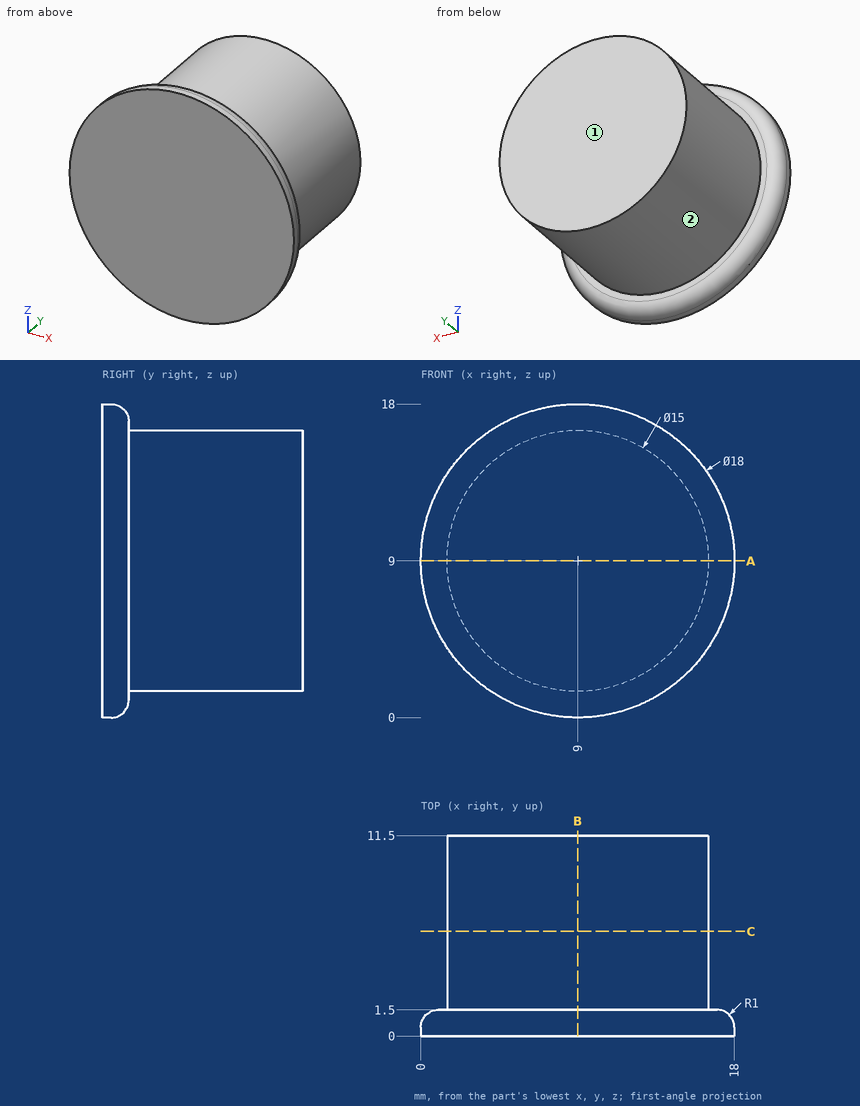
Check sheet for the drawn part. Datum: minimum x, y, z corner. Units: mm. A direction names the side the tool comes from. Round coordinates to 2 decimals unless told otherwise and drop trailing zeros. Write each loop counter-clockwise with the first axis right and the second up, starting at its lowest first coordinate (ties: lowest second). Pieces come first, ordered by that corner, then holes. Notation, with made-up numbers: (2, 86.25) -> (36, 86.25) arc R10 cw to (36, 93.25) -> close; hole circle Ø5 at (-6, -30.75). An arc over 180 degrees is marked (long way). One line per item, written item: value. Start each with the question number.
(1) Scan lines: line 1 (Z direction, x = 15.25, y = 3); line 2 (X direction, y = 8.75, z = 13); line 3 (Z direction, x = 4.75, y = 4). Record each from-to range of solid material in increasing order. Write a range as [from, to].
(2) Cross-section at C-C, the plane y = 6. Record the cut outline in (x, z).
(3) Go/stop test with flat-tipped pins: pin 1 Ø2 at (y, z) = (1.5, 13) entering from +X; pin 2 Ø1 at (y, z) = (6, 4) entering from +X; pin 3 Ø1.5 at (y, z) = (6, 2) entering from +X. Record where each tip stops, or that it passes through.
(4) Cross-section at B-B, the plane x = 9. Record the cut outline in (y, z), and give its area (3 significant figures).
(5) Access from +Z, -Z, +X, -X, +Y, -Y to the whole of each face (thin tool, end or side, straight path). Record for the marked faces 1 and 2.
(6) Cross-section at A-A, the plane z = 9. Record the cut outline in (x, y), and give its area (3 significant figures).
Answer:
1. line 1: [4.85, 13.15]
1. line 2: [2.66, 15.34]
1. line 3: [2.82, 15.18]
2. outline: circle Ø15 at (9, 9)
3. pin 1: x = 17.33
3. pin 2: x = 15
3. pin 3: x = 13.15
4. outline: (0, 0) -> (0.5, 0) arc R1 ccw to (1.5, 1) -> (1.5, 1.5) -> (11.5, 1.5) -> (11.5, 16.5) -> (1.5, 16.5) -> (1.5, 17) arc R1 ccw to (0.5, 18) -> (0, 18) -> close
4. area: 177 mm²
5. face 1: +Z, -Z, +X, -X, +Y
5. face 2: +Y
6. outline: (0, 0) -> (18, 0) -> (18, 0.5) arc R1 ccw to (17, 1.5) -> (16.5, 1.5) -> (16.5, 11.5) -> (1.5, 11.5) -> (1.5, 1.5) -> (1, 1.5) arc R1 ccw to (0, 0.5) -> close
6. area: 177 mm²
